Can you work these out from the drawing? Everything is in mm from the part's minimum corner. Give positions to 0.01 mm unless a question says otherwise; leave off trailing zeros. Order: outer loops, then holes, each group sorted by start corner. A loop starts at its lowest first (then second) coordinate and runs counter-clockwise, first axis right, second up. Notation, with made-up numbers: (-16, -7) -> (9, -7) arc R15 ccw to (9, 21) -> close; hole circle Ø2 at (16.25, -23.5). An arc over 180 degrees is marked (long way). One line per item, written item: value.
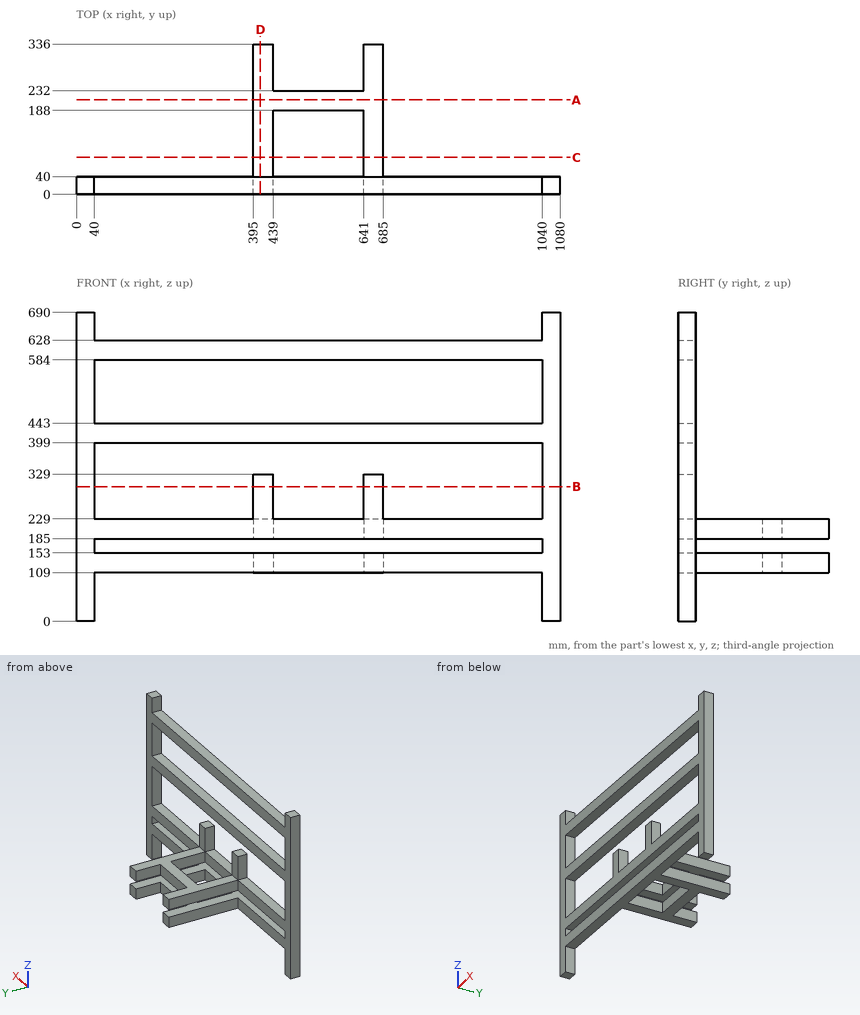
1) Suppose I cut it at D-D, the plane x = 410.5. Write out the boundary of the cut face in (y, z).
Answer below:
outline: (0, 109) -> (336, 109) -> (336, 153) -> (0, 153) -> close; (0, 185) -> (336, 185) -> (336, 229) -> (40, 229) -> (40, 329) -> (0, 329) -> close; (0, 399) -> (40, 399) -> (40, 443) -> (0, 443) -> close; (0, 584) -> (40, 584) -> (40, 628) -> (0, 628) -> close
2) Suppose I cut it at A-A, the plane y = 211. Write out the boundary of the cut face in (x, z).
Answer below:
outline: (395, 109) -> (685, 109) -> (685, 153) -> (395, 153) -> close; (395, 185) -> (685, 185) -> (685, 229) -> (395, 229) -> close
3) If I drill on line 1 along X through (y, z) = (261.5, 122); line 2 along Z through (x, y) = (606.5, 230.5); line 3 along Y through (x, z) = (559, 618.5), over which ranges is the centre line in solid material (lowest first)?
Answer below:
line 1: x = 395 to 439, 641 to 685
line 2: z = 109 to 153, 185 to 229
line 3: y = 0 to 40
4) Suppose I cut it at B-B, the plane z = 301. Write out the boundary of the cut face in (x, y).
Answer below:
outline: (0, 0) -> (40, 0) -> (40, 40) -> (0, 40) -> close; (395, 0) -> (439, 0) -> (439, 40) -> (395, 40) -> close; (641, 0) -> (685, 0) -> (685, 40) -> (641, 40) -> close; (1040, 0) -> (1080, 0) -> (1080, 40) -> (1040, 40) -> close
5) For P1, Ø13, axis at x = 424, z = 261, coming from the +Y side; P2, Ø12, axis at x = 423.5, y = 11, coming from the +Z side, each with a flat end and sliding along its axis, tell me the tip position at first contact or that it passes through.
Answer below:
P1: stops at y = 40
P2: stops at z = 628
6) Suppose I cut it at C-C, the plane y = 83. Write out the boundary of the cut face in (x, z), then the cut area to 3 significant figures.
Answer below:
outline: (395, 109) -> (439, 109) -> (439, 153) -> (395, 153) -> close; (395, 185) -> (439, 185) -> (439, 229) -> (395, 229) -> close; (641, 109) -> (685, 109) -> (685, 153) -> (641, 153) -> close; (641, 185) -> (685, 185) -> (685, 229) -> (641, 229) -> close
area: 7,740 mm2
